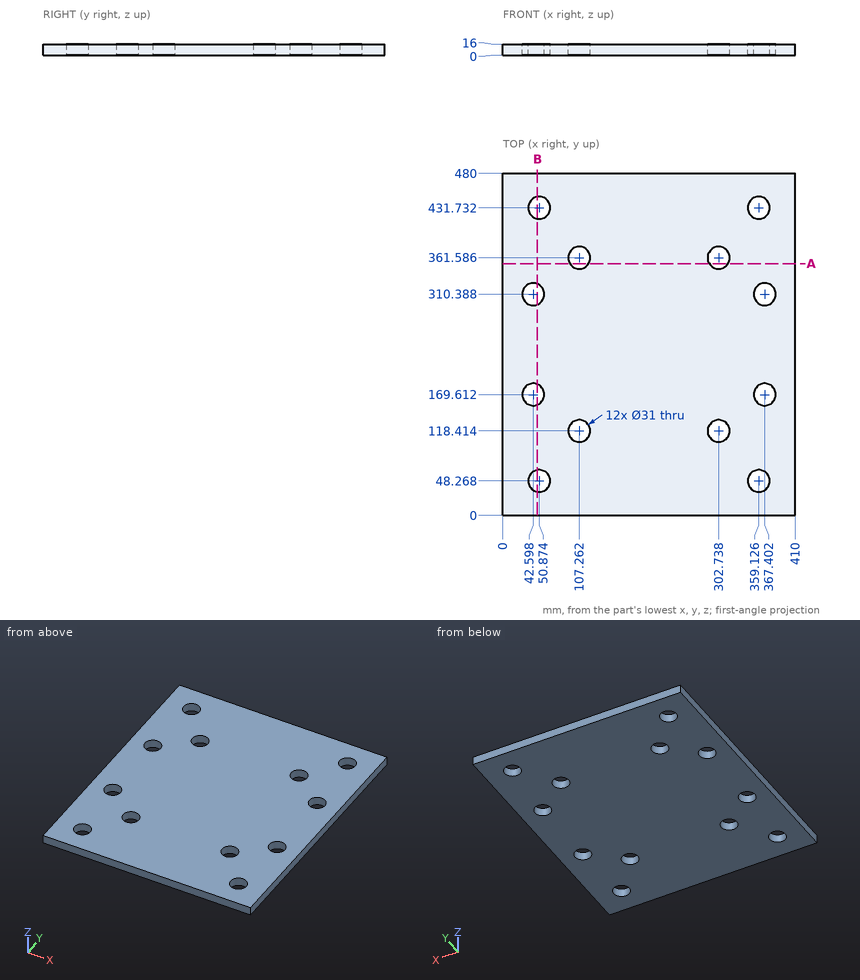
Geometry: see drawing. Coordinates: mm, zero at the bounding-box minimum. Coordinates: 2 decimals unless noted, no trailing zeros. Loops run counter-clockwise (first coordinate to the right, second up) from the corner with the lowest first, then second, coordinate; pieces in that order, holes last. Notation, with made-up numbers: M -10,12 L 6,12 A10 cw 6,28 Z; hole C 44.5,70 d1. An arc over 180 degrees is marked long. Put each result on its own line as item: value. Start each with the question number.
1) Contact query for a flat-ended pin moving along its axis: pin 1 Ø18.5 at (x, y) = (42.6, 169.61) entering from -Z. Output: stop coordinate, or through.
2) Ray query, L1, parallel to X at y = 297, z = 11.75 (1 decimal); L2, parallel to Y at x = 302, z = 4.75; L3, parallel to X at y = 364.5, z = 10.5 (1 decimal). Return the intervals inside material, ascending. Write a range as from..to.
3) Cut plane B-B on x = 48.5. Give the number of separate pieces and of enclosed holes in the cut face, then the cut area to 3 significant figures.
4) Cut plane A-A on y = 353.5. Return the cut outline in (x, z) (1 decimal), then the cut area to 3 significant figures.
The answers:
1. pin 1: passes through
2. L1: x = 0..34.8, 50.4..359.6, 375.2..410
2. L2: y = 0..102.93, 133.9..346.1, 377.07..480
2. L3: x = 0..92, 122.5..287.5, 318..410
3. separate pieces: 5
3. enclosed holes: 0
3. area: 5,780 mm²
4. outline: M 0,0 L 94,0 L 94,16 L 0,16 Z; M 120.5,0 L 289.5,0 L 289.5,16 L 120.5,16 Z; M 316,0 L 410,0 L 410,16 L 316,16 Z
4. area: 5,710 mm²
